Verification items for the finished model (mm, model axes). Give positions to 0.01 mm unless a question says otherwise; leave off trailing zeros. Loops run counter-clockwise (first coordinate to the right, second up) from the corner with the lowest first, then second, coordinate; pieces in that order, holes last. Notation, with made-up numbers: (66.5, 29.5) - (117.5, 29.5) arc R17 ccw to (117.5, 43.5) - close; hole circle Ø7 at (74.25, 32). An arc over 180 degrees is marked (long way). Answer in a Markdown table with one row per item.
```python
from build123d import *

# Parameters (mm, degrees)
SKETCH1_W               = 128
SKETCH1_H               = 41
BOSS_EXTRUDE1_DEPTH     = 3
CUT_EXTRUDE2_START      = -4
CUT_EXTRUDE2_DEPTH      = 5
LPATTERN3_COUNT         = 12
LPATTERN3_PITCH         = 10
CUT_EXTRUDE3_START      = -4
CUT_EXTRUDE3_DEPTH      = 5
LPATTERN5_COUNT         = 12
LPATTERN5_PITCH         = 10
CUT_EXTRUDE4_START      = -4
SKETCH6_R               = 1.6
CUT_EXTRUDE4_DEPTH      = 5
MIRROR3_START           = -4
MIRROR3_COPY_1_SKETCH_R = 1.6
MIRROR3_COPY_1_DEPTH    = 5
CUT_EXTRUDE5_START      = -4
CUT_EXTRUDE5_DEPTH      = 5
CUT_EXTRUDE6_START      = -4
SKETCH8_W               = 4
SKETCH8_H               = 10
CUT_EXTRUDE6_DEPTH      = 5


with BuildPart() as part:
    # Sketch1 → Boss-Extrude1 (new body)
    with BuildSketch(Plane(origin=(0, 0, 0), x_dir=(1, 0, 0), z_dir=(0, 1, 0))):
        Rectangle(SKETCH1_W, SKETCH1_H)
    extrude(amount=BOSS_EXTRUDE1_DEPTH)

    # Sketch2 → Cut-Extrude2 (cut)
    with BuildSketch(Plane(origin=(0, 3, 0), x_dir=(1, 0, 0), z_dir=(0, 1, 0)).offset(CUT_EXTRUDE2_START)):
        Polygon((-60, 20.5), (-55, 10.5), (-50, 20.5), align=None)
    cut_extrude2 = extrude(amount=CUT_EXTRUDE2_DEPTH, mode=Mode.SUBTRACT)

    # LPattern3: Cut-Extrude2 ×12
    with Locations(*[(i * LPATTERN3_PITCH, 0, 0) for i in range(1, LPATTERN3_COUNT)]):
        add(cut_extrude2, mode=Mode.SUBTRACT)

    # Sketch5 → Cut-Extrude3 (cut)
    with BuildSketch(Plane(origin=(0, 3, 0), x_dir=(1, 0, 0), z_dir=(0, 1, 0)).offset(CUT_EXTRUDE3_START)):
        Polygon((-55, -20.5), (-60, -10.5), (-60, -20.5), align=None)
        Polygon((-50, -10.5), (-55, -20.5), (-50, -20.5), align=None)
    cut_extrude3 = extrude(amount=CUT_EXTRUDE3_DEPTH, mode=Mode.SUBTRACT)

    # LPattern5: Cut-Extrude3 ×12
    with Locations(*[(i * LPATTERN5_PITCH, 0, 0) for i in range(1, LPATTERN5_COUNT)]):
        add(cut_extrude3, mode=Mode.SUBTRACT)

    # Sketch6 → Cut-Extrude4 (cut)
    with BuildSketch(Plane(origin=(0, 3, 0), x_dir=(1, 0, 0), z_dir=(0, 1, 0)).offset(CUT_EXTRUDE4_START)):
        with Locations((-58.5, 4.5)):
            Circle(SKETCH6_R)
    cut_extrude4 = extrude(amount=CUT_EXTRUDE4_DEPTH, mode=Mode.SUBTRACT)

    # Mirror2: Cut-Extrude4 across plane
    add(cut_extrude4.mirror(Plane(origin=(0, 0, 0), x_dir=(0, 0, 1), z_dir=(1, 0, 0))), mode=Mode.SUBTRACT)

    # Mirror3: Cut-Extrude4 across plane
    add(cut_extrude4.mirror(Plane.XY), mode=Mode.SUBTRACT)

    # Mirror3 copy 1 sketch → Mirror3 copy 1 (cut)
    with BuildSketch(Plane(origin=(0, 3, 0), x_dir=(-1, 0, 0), z_dir=(0, 1, 0)).offset(MIRROR3_START)):
        with Locations((-58.5, 4.5)):
            Circle(MIRROR3_COPY_1_SKETCH_R)
    extrude(amount=MIRROR3_COPY_1_DEPTH, mode=Mode.SUBTRACT)

    # Sketch7 → Cut-Extrude5 (cut)
    with BuildSketch(Plane(origin=(0, 3, 0), x_dir=(1, 0, 0), z_dir=(0, 1, 0)).offset(CUT_EXTRUDE5_START)):
        Polygon((-60, 20.5), (-64, 10.5), (-64, 20.5), align=None)
    cut_extrude5 = extrude(amount=CUT_EXTRUDE5_DEPTH, mode=Mode.SUBTRACT)

    # Mirror4: Cut-Extrude5 across plane
    add(cut_extrude5.mirror(Plane(origin=(0, 0, 0), x_dir=(0, 0, 1), z_dir=(1, 0, 0))), mode=Mode.SUBTRACT)

    # Sketch8 → Cut-Extrude6 (cut)
    with BuildSketch(Plane(origin=(0, 3, 0), x_dir=(1, 0, 0), z_dir=(0, 1, 0)).offset(CUT_EXTRUDE6_START)):
        with Locations((-62, -15.5)):
            Rectangle(SKETCH8_W, SKETCH8_H)
    cut_extrude6 = extrude(amount=CUT_EXTRUDE6_DEPTH, mode=Mode.SUBTRACT)

    # Mirror5: Cut-Extrude6 across plane
    add(cut_extrude6.mirror(Plane(origin=(0, 0, 0), x_dir=(0, 0, 1), z_dir=(1, 0, 0))), mode=Mode.SUBTRACT)


solid = part.part
```
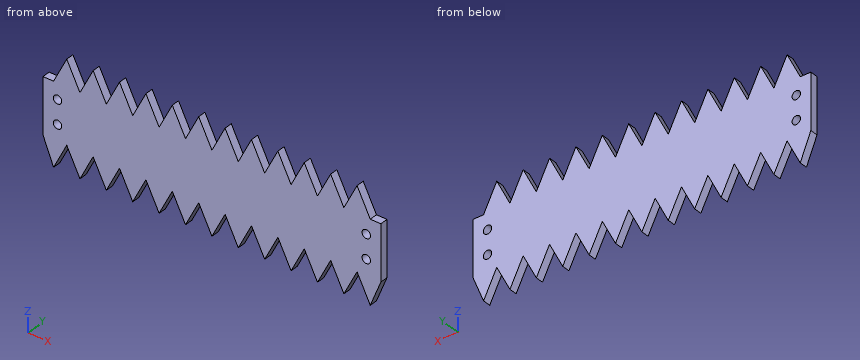
Q1. Sectioned sample at C-C (z = -16.5). Give the number of separate pieces and of enclosed holes in the cut face, and give its area (3 significant figures).
Completed:
| item | result |
|---|---|
| separate pieces | 13 |
| enclosed holes | 0 |
| area | 154 mm^2 |
Q2. Go/stop test with flat-tipped pins: P1, Ø1.9, axis at x = -58.5, z = 4.5, coming from the -Y side; P2, Ø0.9, axis at x = -62.5, y = 1, coming from the +Z side. Record where each tip stops, or that it passes through.
Completed:
| item | result |
|---|---|
| P1 | through |
| P2 | z = 10.5 |
Q3. Sectioned sample at A-A (x = -58.5). Record the cut outline in (y, z).
Completed:
| item | result |
|---|---|
| outline | (0, -17.5) - (3, -17.5) - (3, -6.1) - (0, -6.1) - close; (0, -2.9) - (3, -2.9) - (3, 2.9) - (0, 2.9) - close; (0, 6.1) - (3, 6.1) - (3, 13.5) - (0, 13.5) - close |
Q4. Sectioned sample at B-B (z = -4.5). Record the cut outline in (x, y).
Completed:
| item | result |
|---|---|
| outline | (-64, 0) - (-60.1, 0) - (-60.1, 3) - (-64, 3) - close; (-56.9, 0) - (56.9, 0) - (56.9, 3) - (-56.9, 3) - close; (60.1, 0) - (64, 0) - (64, 3) - (60.1, 3) - close |
Q5. Thickness scan on line 1 (Z direction, x = 58.5, y = 2.25); line 2 (X direction, y = 1.5, z = 5); line 3 (X direction, y = 2.2, z = 5.5). Record the ranges inside material, lowest first.
Completed:
| item | result |
|---|---|
| line 1 | -17.5 to -6.1, -2.9 to 2.9, 6.1 to 13.5 |
| line 2 | -64 to -60.02, -56.98 to 56.98, 60.02 to 64 |
| line 3 | -64 to -59.75, -57.25 to 57.25, 59.75 to 64 |
